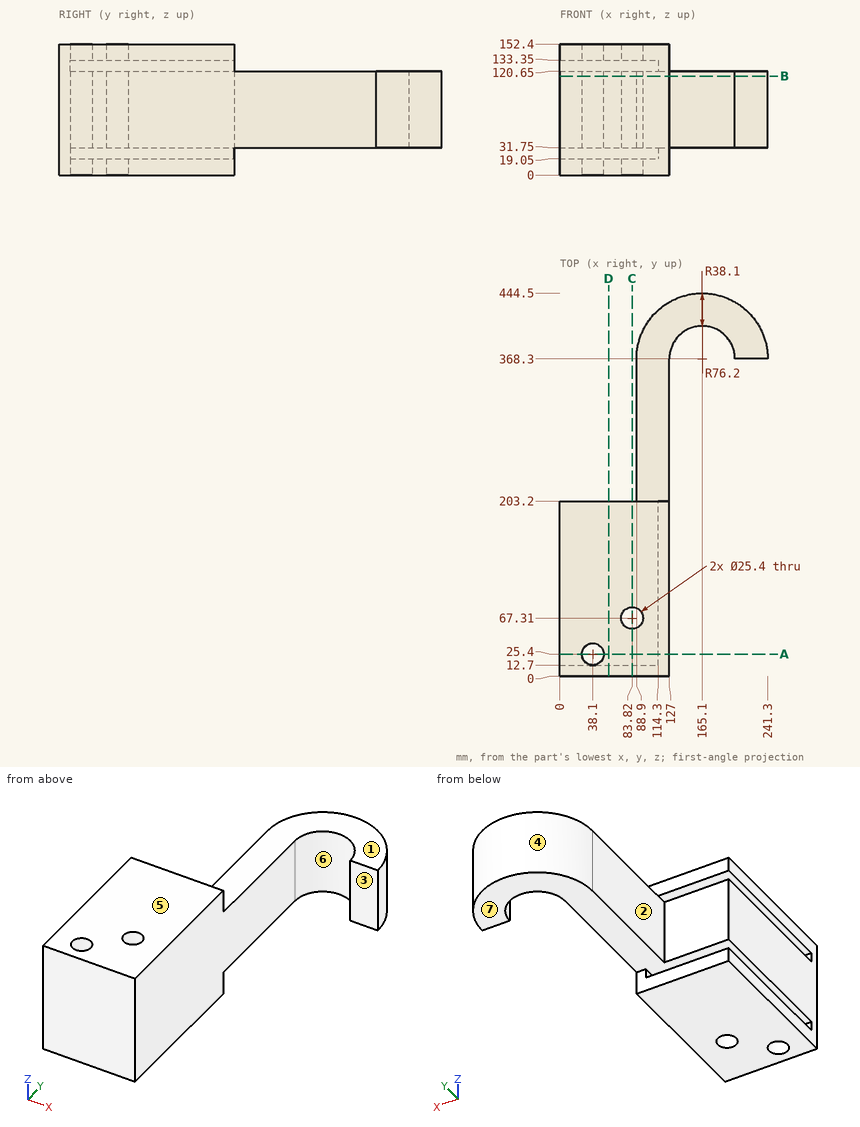
The figure shows three views and two pictorial views of one solid part (mm, origin at its lowest corner). Answer the questions. A direction names the side the tool comes from. Give positions to 0.01 mm unless a question says otherwise; leave off trailing zeros. Write each loop counter-clockwise with the first axis right and the second up, starting at its lowest first coordinate (ties: lowest second). Pieces come first, ordered by that corner, then holes.
Q1. The part is cut by section C-C on x = 83.82. Give the vertices of the cut face in (y, z), and give its area (3 significant figures).
Answer:
outline: (0, 0) - (54.61, 0) - (54.61, 19.05) - (12.7, 19.05) - (12.7, 31.75) - (54.61, 31.75) - (54.61, 120.65) - (12.7, 120.65) - (12.7, 133.35) - (54.61, 133.35) - (54.61, 152.4) - (0, 152.4) - close; (80.01, 0) - (203.2, 0) - (203.2, 19.05) - (80.01, 19.05) - close; (80.01, 31.75) - (203.2, 31.75) - (203.2, 120.65) - (80.01, 120.65) - close; (80.01, 133.35) - (203.2, 133.35) - (203.2, 152.4) - (80.01, 152.4) - close
area: 22,900 mm2
Q2. Straight lines are drawn through the part: L1, parallel to Z at x = 47, y = 53.5; L2, parallel to X at y = 67.31, z = 140.25; L3, parallel to Y at x = 83.82, z = 5.5. For each, find the intervals that lie inside material, in ascending order.
Answer:
L1: z = 0 to 19.05, 31.75 to 120.65, 133.35 to 152.4
L2: x = 0 to 71.12, 96.52 to 127
L3: y = 0 to 54.61, 80.01 to 203.2
Q3. The part is cut by section A-A on y = 25.4. Give the vertices of the cut face in (x, z).
Answer:
outline: (0, 0) - (25.4, 0) - (25.4, 19.05) - (0, 19.05) - close; (0, 31.75) - (25.4, 31.75) - (25.4, 120.65) - (0, 120.65) - close; (0, 133.35) - (25.4, 133.35) - (25.4, 152.4) - (0, 152.4) - close; (50.8, 0) - (127, 0) - (127, 152.4) - (50.8, 152.4) - (50.8, 133.35) - (114.3, 133.35) - (114.3, 120.65) - (50.8, 120.65) - (50.8, 31.75) - (114.3, 31.75) - (114.3, 19.05) - (50.8, 19.05) - close
Q4. For a pull along Z with two mould halves and no side action, classify the marked faces 5, 6 and 7 as released by +Z, released by -Z, zero draft, split by the parting line, or undercut.
Answer:
face 5: released by +Z
face 6: zero draft
face 7: undercut
Q5. The part is cut by section D-D on x = 56.5. Give the vertices of the cut face in (y, z), and give its area (3 significant figures).
Answer:
outline: (0, 0) - (203.2, 0) - (203.2, 19.05) - (12.7, 19.05) - (12.7, 31.75) - (203.2, 31.75) - (203.2, 120.65) - (12.7, 120.65) - (12.7, 133.35) - (203.2, 133.35) - (203.2, 152.4) - (0, 152.4) - close
area: 26,100 mm2
Q6. The part is cut by section B-B on z = 115. Give the vertices of the cut face in (x, y).
Answer:
outline: (0, 0) - (127, 0) - (127, 368.3) arc R38.1 cw to (203.2, 368.3) - (241.3, 368.3) arc R76.2 ccw to (88.9, 368.3) - (88.9, 203.2) - (0, 203.2) - close; hole circle Ø25.4 at (38.1, 25.4); hole circle Ø25.4 at (83.82, 67.31)
Q7. A tool of negligible diameter and unlimited length cuts with its end or side. For the marked faces 1, 2, 3 and 4, from which of +Z, -Z, +X, -X, +Y, -Y can it reach the whole face along a straight path? Write none if from no direction.
Answer:
face 1: -X, +Y
face 2: +Z, -Z, -X, +Y
face 3: +Z, -Z, +X, -Y
face 4: +Z, -Z, +Y
Q8. Given pin 1 (10 mm diameter, centred on x = 186, z = 117.5, fed in from +Y); pin 2 (20.5 mm diameter, centred on x = 83.82, y = 67.31, fed in from +Z); pin 3 (10 mm diameter, centred on y = 87.5, z = 25, fed in from -X); pin 4 (12 mm diameter, centred on x = 213.5, z = 61.5, fed in from -Y), each flat-ended and moving along its own axis, determine where each tip first touches the part or whether it passes through.
Answer:
pin 1: stops at y = 442.82
pin 2: passes through
pin 3: stops at x = 114.3
pin 4: stops at y = 368.3
